Drawing for the job (mm, zero at the part's lowest x, y, z). Give positions to 0.01 mm unless a question says otherwise; leave off trailing zeros. Order: outer loops, then holes, each group sorted by start corner. A loop starts at its lowest first (then second) coordinate and runs counter-clockwise, first axis right, second up. Notation, with made-up numbers: (50.5, 72.5) - (75.5, 72.5) arc R4 ccw to (75.5, 77.5) - close; hole circle Ø6 at (-6.5, 67.25). An arc over 180 degrees is marked (long way). Use a Markdown table: item, result.
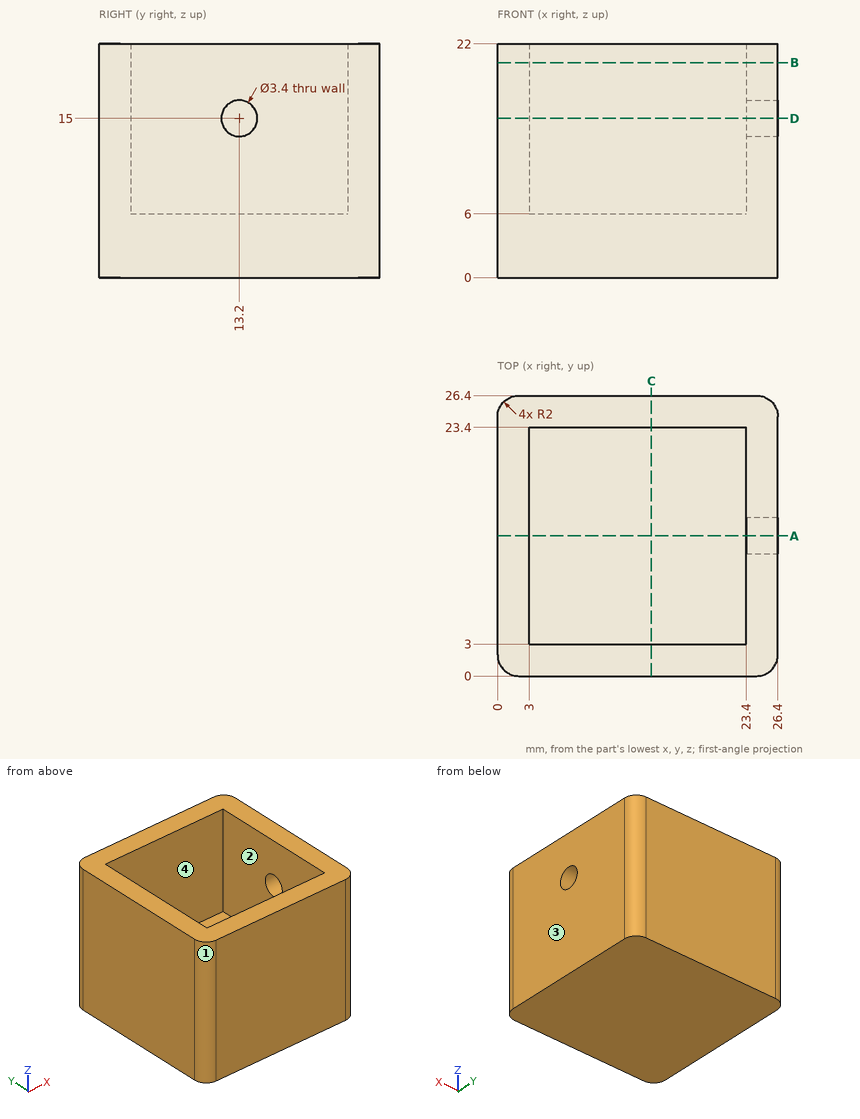
1) Wall check: line 1 (X direction, y = 21.5, z = 9); line 2 (Z direction, x = 25.7, y = 13.2). Give the ranges that are in metal, low to high. Write a range as from..to.
Computed:
| item | result |
|---|---|
| line 1 | x = 0..3, 23.4..26.4 |
| line 2 | z = 0..13.3, 16.7..22 |
2) Slice it at B-B (z = 20.25). Write the cut outline in (x, y).
Computed:
| item | result |
|---|---|
| outline | (0, 2) arc R2 ccw to (2, 0) - (24.4, 0) arc R2 ccw to (26.4, 2) - (26.4, 24.4) arc R2 ccw to (24.4, 26.4) - (2, 26.4) arc R2 ccw to (0, 24.4) - close; hole (3, 3) - (23.4, 3) - (23.4, 23.4) - (3, 23.4) - close |
3) Slice it at D-D (z = 15). Write the cut outline in (x, y).
Computed:
| item | result |
|---|---|
| outline | (0, 2) arc R2 ccw to (2, 0) - (24.4, 0) arc R2 ccw to (26.4, 2) - (26.4, 11.5) - (23.4, 11.5) - (23.4, 3) - (3, 3) - (3, 23.4) - (23.4, 23.4) - (23.4, 14.9) - (26.4, 14.9) - (26.4, 24.4) arc R2 ccw to (24.4, 26.4) - (2, 26.4) arc R2 ccw to (0, 24.4) - close |
4) Slice it at C-C (x = 14.5). Write the cut outline in (y, z), and give its area (3 significant figures).
Computed:
| item | result |
|---|---|
| outline | (0, 0) - (26.4, 0) - (26.4, 22) - (23.4, 22) - (23.4, 6) - (3, 6) - (3, 22) - (0, 22) - close |
| area | 254 mm² |
5) Two-plate mould, pull along X, no slides. Class the marked faces 1, 2, 3 and 4: +X half, -X half, draft (parallel to the pull), parting line (faces both ways), or undercut.
Computed:
| item | result |
|---|---|
| face 1 | -X half |
| face 2 | undercut |
| face 3 | +X half |
| face 4 | undercut |
6) Slice it at A-A (y = 13.2). Write the cut outline in (x, z), and give its area (3 significant figures).
Computed:
| item | result |
|---|---|
| outline | (0, 0) - (26.4, 0) - (26.4, 13.3) - (23.4, 13.3) - (23.4, 6) - (3, 6) - (3, 22) - (0, 22) - close; (23.4, 16.7) - (26.4, 16.7) - (26.4, 22) - (23.4, 22) - close |
| area | 244 mm² |
